```python
from build123d import *

# Parameters (mm, degrees)
SKETCH1_W               = 76.2
SKETCH1_H               = 50.8
SKETCH1_R               = 14.2748
BOSS_EXTRUDE1_DEPTH     = 3.175
SKETCH2_R               = 22.225
BOSS_EXTRUDE2_DEPTH     = 4.445
SKETCH3_R               = 14.2748
CUT_EXTRUDE1_DEPTH      = 92.688810795
SKETCH4_R               = 15.8623
CUT_EXTRUDE2_DEPTH      = 1.6002
FILLET2_R               = 2.54
CUT_EXTRUDE3_DEPTH      = 92.688810795
CUT_EXTRUDE3_DEPTH_BACK = 92.688810795
SKETCH5_R               = 2.54
CUT_EXTRUDE4_DEPTH      = 92.688810795
SKETCH7_R               = 4.699
CUT_EXTRUDE5_DEPTH      = 92.688810795
SKETCH9_R               = 4.699
CUT_EXTRUDE6_DEPTH      = 92.688810795


with BuildPart() as part:
    # Sketch1 → Boss-Extrude1 (new body)
    with BuildSketch(Plane(origin=(0, 0, 0), x_dir=(1, 0, 0), z_dir=(0, 1, 0))):
        with Locations((38.1, 25.4)):
            Rectangle(SKETCH1_W, SKETCH1_H)
        with Locations(Location((38.1, 25.4, 0), (0, 0, 270))):
            Circle(SKETCH1_R, mode=Mode.SUBTRACT)
    extrude(amount=BOSS_EXTRUDE1_DEPTH)

    # Sketch2 → Boss-Extrude2 (add)
    with BuildSketch(Plane(origin=(0, 3.175, 0), x_dir=(1, 0, 0), z_dir=(0, 1, 0))):
        with Locations(Location((38.1, 25.4, 0), (0, 0, 90))):
            Circle(SKETCH2_R)
    extrude(amount=BOSS_EXTRUDE2_DEPTH)

    # Sketch3 → Cut-Extrude1 (cut, through all)
    with BuildSketch(Plane.XZ.offset(-3.175)):
        with Locations(Location((38.1, -25.4, 0), (0, 0, 270))):
            Circle(SKETCH3_R)
    extrude(amount=-CUT_EXTRUDE1_DEPTH, mode=Mode.SUBTRACT)

    # Sketch4 → Cut-Extrude2 (cut)
    with BuildSketch(Plane(origin=(0, 0, 0), x_dir=(-1, 0, 0), z_dir=(0, -1, 0))):
        with Locations(Location((-38.332507849, 25.4, 0), (0, 0, 90))):
            Circle(SKETCH4_R)
    extrude(amount=-CUT_EXTRUDE2_DEPTH, mode=Mode.SUBTRACT)

    # Fillet2
    fillet2_edges = [part.edges().sort_by_distance(p)[0] for p in [
        (0, 1.5875, -50.8),
        (76.2, 1.5875, -50.8),
        (76.2, 1.5875, 0),
        (0, 1.5875, 0),
    ]]
    fillet(fillet2_edges, radius=FILLET2_R)

    # Sketch5 → Cut-Extrude3 (cut, two sides: drawn at the far end of the back side and taken through both)
    with BuildSketch(Plane(origin=(0, 3.175, 0), x_dir=(1, 0, 0), z_dir=(0, 1, 0)).offset(-CUT_EXTRUDE3_DEPTH_BACK)):
        with Locations(Location((69.85, 41.275, 0), (0, 0, 270))):
            Circle(SKETCH5_R)
        with Locations(Location((69.85, 9.525, 0), (0, 0, 270))):
            Circle(SKETCH5_R)
        with Locations(Location((19.05, 9.525, 0), (0, 0, 270))):
            Circle(SKETCH5_R)
        with Locations(Location((19.05, 41.275, 0), (0, 0, 270))):
            Circle(SKETCH5_R)
    extrude(amount=CUT_EXTRUDE3_DEPTH + CUT_EXTRUDE3_DEPTH_BACK, mode=Mode.SUBTRACT)

    # Sketch6 → Cut-Extrude4 (cut, through all)
    with BuildSketch(Plane(origin=(0, 3.175, 0), x_dir=(1, 0, 0), z_dir=(0, 1, 0))):
        with BuildLine():
            Line((0, 48.26), (0, 2.54))
            ThreePointArc((0, 2.54), (0.743948776, 0.743948776), (2.54, 0))
            Line((2.54, 0), (25.399999995, 0))
            ThreePointArc((25.399999995, 0), (11.359611147, 9.31110396), (6.233986574, 25.359691084))
            ThreePointArc((6.233986574, 25.359691084), (11.333824667, 41.457338196), (25.399999042, 50.8))
            Line((25.399999042, 50.8), (2.54, 50.8))
            ThreePointArc((2.54, 50.8), (0.743948776, 50.056051224), (0, 48.26))
        make_face()
    extrude(amount=-CUT_EXTRUDE4_DEPTH, mode=Mode.SUBTRACT)

    # Sketch7 → Cut-Extrude5 (cut, through all)
    with BuildSketch(Plane(origin=(0, 3.175, 0), x_dir=(1, 0, 0), z_dir=(0, 1, 0))):
        with Locations((19.05, 9.525)):
            Circle(SKETCH7_R)
    extrude(amount=CUT_EXTRUDE5_DEPTH, mode=Mode.SUBTRACT)

    # Sketch9 → Cut-Extrude6 (cut, through all)
    with BuildSketch(Plane(origin=(0, 3.175, 0), x_dir=(1, 0, 0), z_dir=(0, 1, 0))):
        with Locations((19.05, 41.275)):
            Circle(SKETCH9_R)
    extrude(amount=CUT_EXTRUDE6_DEPTH, mode=Mode.SUBTRACT)


solid = part.part
```
The listing builds one solid part. Answer for the finished solid, in the listing's coordinates (mm). A direction names the side the tool comes from. Give positions to 0.01 mm unless a question says otherwise; leave off trailing zeros. Write each loop counter-clockwise with the first axis right and the second up, starting at its lowest first coordinate (ties: lowest second). Pieces come first, ordered by that corner, then holes. Notation, with made-up numbers: M 82.25,60.25 L 106.25,60.25 A24 ccw 106.25,86.25 Z; hole C 26.25,63.5 d8. An arc over 180 degrees is marked long. Write each question's results on one line, items separated by ' | '.
Q1. Section B-B, the plane y = 6.5 is taken. Write down the section's boundary in (x, z) (3 decimals).
Output values:
outline: M 18.891,-36.579 A4.699 cw 23.641,-42.278 A22.225 ccw long 23.641,-8.522 A4.699 cw 18.891,-14.221 A22.225 ccw Z; hole C 38.1,-25.4 d28.55
Q2. Section C-C, the plane z = -31 is taken. Write down the section's boundary in (x, y) (1 decimal).
Output values:
outline: M 6.7,0 L 23.5,0 L 23.5,1.6 L 25,1.6 L 25,7.6 L 16.6,7.6 L 16.6,3.2 L 6.7,3.2 Z; M 51.2,1.6 L 53.2,1.6 L 53.2,0 L 76.2,0 L 76.2,3.2 L 59.6,3.2 L 59.6,7.6 L 51.2,7.6 Z
Q3. Flat-ended cylindrical pins translate along their axes: P1, Ø1, axis at x = 52.5, y = 6.5, coming from the -Z side; P2, Ø3, axis at x = 19.05, z = -9.525, coming from the -Y side; P3, Ø6, axis at x = 19.05, z = -41.275, coming from the +Y side (3 decimals); P4, Ø1.5, axis at y = 4.5, z = -36, coming from the -X side. Find the tip coordinate at first contact, or state that the pin passes through.
Output values:
P1: z = -42.74 | P2: through | P3: y = 3.175 | P4: x = 18.18
Q4. Section A-A, the plane x = 69.85 is taken. Write down the section's boundary in (y, z) (3 decimals), then the cut area to 3 significant figures.
Output values:
outline: M 0,-50.8 L 3.175,-50.8 L 3.175,-43.815 L 0,-43.815 Z; M 0,-38.735 L 3.175,-38.735 L 3.175,-12.065 L 0,-12.065 Z; M 0,-6.985 L 3.175,-6.985 L 3.175,0 L 0,0 Z | area: 129 mm2
Q5. Consider L1, parallel to Z at x = 19.05, y = 2.15 (3 decimals); L2, parallel to Z at x = 38, y = 6.25; L3, parallel to X at y = 2.4, z = -25.4. Determine where each line is inside the solid, lowest interval first. Write a range as from..to.
Output values:
L1: -48.245..-43.815, -38.735..-12.065, -6.985..-2.556 | L2: -47.62..-39.67, -11.13..-3.18 | L3: 6.23..23.83, 52.37..76.2
Q6. A tool of negligible diameter and unlimited length cuts with its end or side. For faces 5 (the cylindrical face through (15.876, 5.366, -25.564)), 6 (the cylindrical face through (54.06, 0.79, -23.34)), 7 (the cylindrical face through (60.314, 5.366, -24.691)), from which of +Z, -Z, +X, -X, +Y, -Y can it reach the whole face along a straight path? Write none if from no direction.
Output values:
face 5: -X, +Y | face 6: -Y | face 7: +Y
Q7. For a pull along Z with two mould halves and no side action, classify faces 1 (the cylindrical face through (16.57, 1.57, -41.83)), 2 (the cylindrical face through (75.436, 1.61, -50.076)), 3 (the flat face through (76.2, 2, -25)), 4 (the flat face through (53, 1.6, -25)) as released by +Z, released by -Z, zero draft, split by the parting line, or undercut.
Output values:
face 1: undercut | face 2: released by -Z | face 3: zero draft | face 4: undercut
Q8. Section D-D, the plane x = 49.5 is taken. Write down the section's boundary in (y, z) (3 decimals), then the cut area to 3 significant figures.
Output values:
outline: M 0,-50.8 L 3.175,-50.8 L 3.175,-44.479 L 7.62,-44.479 L 7.62,-33.991 L 1.6,-33.991 L 1.6,-36.665 L 0,-36.665 Z; M 0,-14.135 L 1.6,-14.135 L 1.6,-16.809 L 7.62,-16.809 L 7.62,-6.321 L 3.175,-6.321 L 3.175,0 L 0,0 Z | area: 191 mm2
